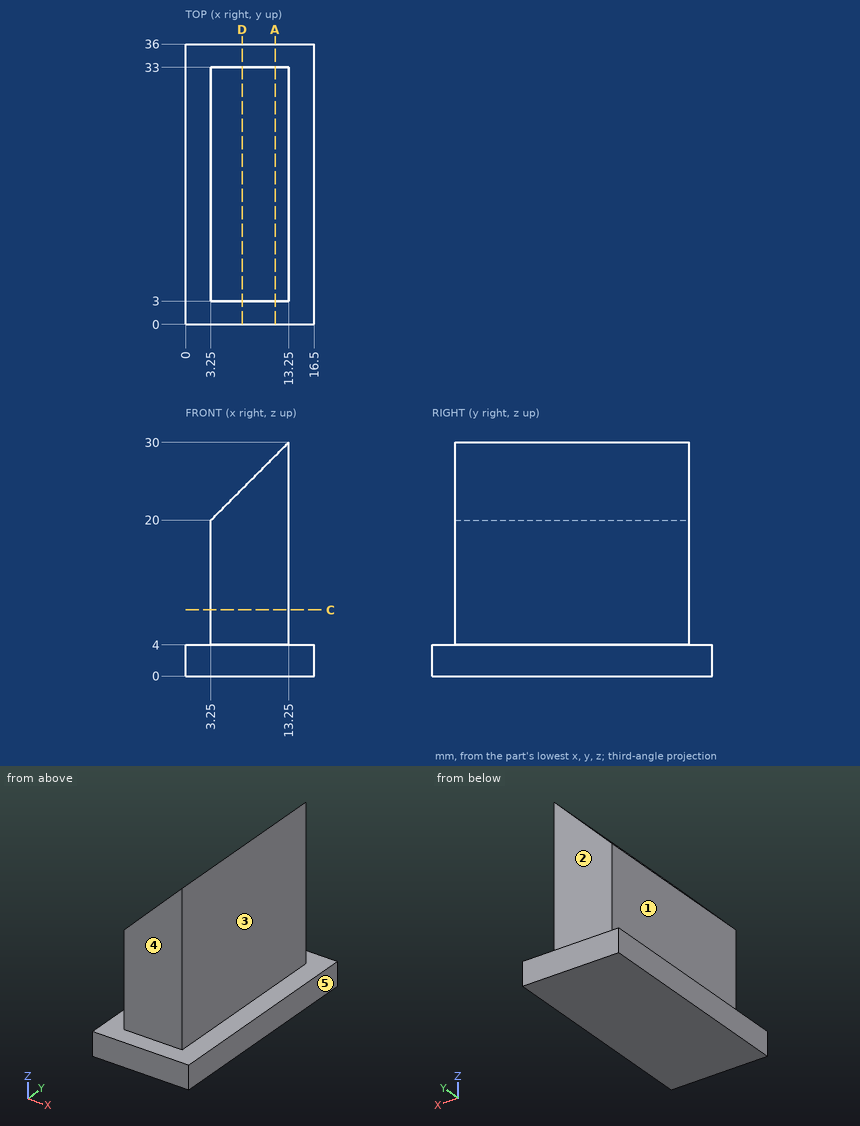
Part print with two shaded views. Sizes in mm from the minimum x, y, z corner. A direction names the side the tool comes from. Round coordinates to 2 decimals unless told otherwise and drop trailing zeros. Order: outer loops, then holes, each group sorted by start corner. A loop starts at its lowest first (then second) coordinate and runs counter-clockwise, first axis right, second up. Notation, with made-up numbers: M 52.5,-12 L 79.5,-12 A28 cw 79.5,26 Z; hole C 9.25,25 d1. An arc over 180 degrees is marked long. Put each result on its own line as item: value. Start each with the question number.
1. Tool access for the marked faces 1, 2, 3, 4 and 5: list every direction of +Z, -Z, +X, -X, +Y, -Y with a clear straight run to the whole face (end or side of a thin tool).
2. Drop flat-ended pins along their axis: pin 1 (8 mm diameter, centred on y = 11, z = 9.5, fed in from -X); pin 2 (5 mm diameter, centred on x = 7.5, z = 7, fed in from +Y); pin 3 (8 mm diameter, centred on y = 5, z = 20.5, fed in from +X). Give the stop position or say it passes through.
3. Slice it at A-A on x = 11.5. List the corners of the cut face in (y, z).
4. Slice it at C-C on z = 8.5. List the corners of the cut face in (x, y), then the cut area to 3 significant figures.
5. Drill centre lines: probe 1 along Z at (x, y) = (14, 15.5); probe 2 along Y at (x, z) = (13, 8.75); probe 3 along X at (y, z) = (19, 9.75). Where is each one in solid material? Low to high. Write a range as [from, to].
6. Slice it at D-D on x = 7.25. List the corners of the cut face in (y, z), then the cut area to 3 significant figures.
Findings:
1. face 1: +Z, -X, +Y, -Y
1. face 2: +Z, +X, -X, +Y
1. face 3: +Z, +X, +Y, -Y
1. face 4: +Z, +X, -X, -Y
1. face 5: +Z, -Z, +X, +Y, -Y
2. pin 1: x = 3.25
2. pin 2: y = 33
2. pin 3: x = 13.25
3. outline: M 0,0 L 36,0 L 36,4 L 33,4 L 33,28.25 L 3,28.25 L 3,4 L 0,4 Z
4. outline: M 3.25,3 L 13.25,3 L 13.25,33 L 3.25,33 Z
4. area: 300 mm2
5. probe 1: [0, 4]
5. probe 2: [3, 33]
5. probe 3: [3.25, 13.25]
6. outline: M 0,0 L 36,0 L 36,4 L 33,4 L 33,24 L 3,24 L 3,4 L 0,4 Z
6. area: 744 mm2
